from build123d import *

# Parameters (mm, degrees)
BOSS_EXTRUDE1_DEPTH        = 3
F_3_0_3_DIAMETER_HOLE2_D   = 3
CIRPATTERN1_COUNT          = 6
F_4_2_4_2_DIAMETER_HOLE1_D = 4.2
F_3_0_3_DIAMETER_HOLE1_D   = 3
FILLET1_R                  = 15
FILLET2_R                  = 2


with BuildPart() as part:
    # Sketch2 → Boss-Extrude1 (new body)
    with BuildSketch(Plane.XY):
        with BuildLine():
            Line((0, -28), (12, -28))
            Line((12, -28), (12, -14.08012784))
            ThreePointArc((12, -14.08012784), (0, 18.5), (-12, -14.08012784))
            Line((-12, -14.08012784), (-12, -28))
            Line((-12, -28), (0, -28))
        make_face()
        with BuildLine():
            ThreePointArc((-3.049823013, 1.717142857), (0, -3.5), (3.049823013, 1.717142857))
            ThreePointArc((3.049823013, 1.717142857), (0, 13.1), (-3.049823013, 1.717142857))
        make_face(mode=Mode.SUBTRACT)
    extrude(amount=BOSS_EXTRUDE1_DEPTH)

    # 3.0 _3_ Diameter Hole2 (through all)
    with Locations(Plane.XY.offset(3)):
        with Locations((15.5, 0)):
            f_3_0_3_diameter_hole2 = Hole(F_3_0_3_DIAMETER_HOLE2_D / 2)

    # CirPattern1: 3.0 _3_ Diameter Hole2 ×6 about axis
    cirpattern1_axis = Axis((0, 0, 0), (0, 0, 1))
    for i in range(1, CIRPATTERN1_COUNT):
        add(f_3_0_3_diameter_hole2.rotate(cirpattern1_axis, i * 360 / CIRPATTERN1_COUNT), mode=Mode.SUBTRACT)

    # 4.2 _4.2_ Diameter Hole1 (through all)
    with Locations(Plane.XY.offset(3)):
        with Locations((0, -16), (0, -24), (8, -24), (-8, -24)):
            Hole(F_4_2_4_2_DIAMETER_HOLE1_D / 2)

    # 3.0 _3_ Diameter Hole1 (through all)
    with Locations(Plane.XY.offset(3)):
        with Locations((8.5, 0), (-8.5, 0)):
            Hole(F_3_0_3_DIAMETER_HOLE1_D / 2)

    # Fillet1
    fillet1_edges = [part.edges().sort_by_distance(p)[0] for p in [
        (-12, -14.08012784, 1.5),
        (12, -14.08012784, 1.5),
    ]]
    fillet(fillet1_edges, radius=FILLET1_R)

    # Fillet2
    fillet2_edges = [part.edges().sort_by_distance(p)[0] for p in [
        (-12, -28, 1.5),
        (12, -28, 1.5),
    ]]
    fillet(fillet2_edges, radius=FILLET2_R)


solid = part.part
CAD build for the part. Positions are in the model's coordinates, mm. A direction names the side the tool comes from. Round coordinates to 2 decimals unless told otherwise and drop trailing zeros. Write each loop counter-clockwise with the first axis right and the second up, starting at its lowest first coordinate (ties: lowest second). Pieces come first, ordered by that corner, then holes. Notation, with made-up numbers: (61.5, 78) -> (90.5, 78) arc R36 ccw to (90.5, 114) -> close; hole circle Ø8 at (-6, 10.25). An arc over 180 degrees is marked (long way). Answer as a JSON object with one key per item and string values.
(1) Band-saw the part on D-D, the plane z = 2.3. Count the separate pieces of the cut face and the enclosed holes in it, then the cut area to 3 significant figures.
Reported:
{"separate pieces": "1", "enclosed holes": "13", "area": "1,090 mm^2"}
(2) Probe probe 1 along Y at (x, z) = (0, 2.4); probe 2 along Y at (x, z) = (8, 1.8); probe 3 along Y at (x, z) = (-0.5, 1.4). List the from-to ranges inside material, lowest first. Write a range as [from, to].
Reported:
{"probe 1": "y = [-28, -26.1], [-21.9, -18.1], [-13.9, -3.5], [13.1, 18.5]", "probe 2": "y = [-28, -26.1], [-21.9, -14.9], [-11.94, -1.41], [1.41, 11.94], [14.9, 16.68]", "probe 3": "y = [-28, -26.04], [-21.96, -18.04], [-13.96, -3.46], [13.08, 18.49]"}
(3) Band-saw the part on B-B, the plane x = -15.5. List the corners of the cut face in (y, z).
Reported:
{"outline": "(-10.1, 0) -> (-1.5, 0) -> (-1.5, 3) -> (-10.1, 3) -> close; (1.5, 0) -> (10.1, 0) -> (10.1, 3) -> (1.5, 3) -> close"}
(4) Band-saw the part on A-A, the plane y = 0. List the corners of the cut face in (x, z).
Reported:
{"outline": "(-18.5, 0) -> (-17, 0) -> (-17, 3) -> (-18.5, 3) -> close; (-14, 0) -> (-10, 0) -> (-10, 3) -> (-14, 3) -> close; (-7, 0) -> (-3.5, 0) -> (-3.5, 3) -> (-7, 3) -> close; (3.5, 0) -> (7, 0) -> (7, 3) -> (3.5, 3) -> close; (10, 0) -> (14, 0) -> (14, 3) -> (10, 3) -> close; (17, 0) -> (18.5, 0) -> (18.5, 3) -> (17, 3) -> close"}
(5) Two-plate mould, pull along X, no slides. Class faces 1 (the face through (0.57, 18.49, 1.48)), 2 (the face through (0.273, -13.918, 1.479)), 3 (the face through (0, -4, 0)): +X half, -X half, draft (parallel to the pull), parting line (faces both ways), or undercut.
Reported:
{"face 1": "parting line", "face 2": "undercut", "face 3": "draft"}
(6) Which spindle directions (+Z, -Z, +X, -X, +Y, -Y) get a long thin tool onto all of the face, cutting with end or side? Do faces 4 (the face through (-12, -23, 1)), 5 (the face through (-6.452, -22.581, 1.479)), 6 (the face through (12, -23, 1)). Say none if no direction does.
Reported:
{"face 4": "+Z, -Z, -X, -Y", "face 5": "+Z, -Z", "face 6": "+Z, -Z, +X, -Y"}
(7) Band-saw the part on C-C, the plane y = 9. List the corners of the cut face in (x, z).
Reported:
{"outline": "(-16.16, 0) -> (-5.76, 0) -> (-5.76, 3) -> (-16.16, 3) -> close; (5.76, 0) -> (16.16, 0) -> (16.16, 3) -> (5.76, 3) -> close"}
(8) Pin check, flat tips, straight feed: P1, Ø2.5, axis at x = -7.75, y = 13.42, coming from the +Z side; P2, Ø4, axis at x = -15.5, y = 0, coming from the +Z side; P3, Ø0.9, axis at y = -23.5, z = 2, coming from the +X side; P4, Ø1.5, axis at y = 13, z = 0.5, coming from the +X side. Stop position of each tip, or through.
Reported:
{"P1": "passes through", "P2": "stops at z = 3", "P3": "stops at x = 12", "P4": "stops at x = 13.86"}
